Job drawing, mm, ordinate dimensions from the low corner. One solid piece. Round coordinates to 2 decimals unless told otherwise and drop trailing zeros. Order: outer loops, then holes, each group sorted by start corner. A loop starts at its lowest first (then second) coordinate and runs counter-clockwise, first axis right, second up. Notation, with made-up numbers: (-35.75, 55.25) -> (-19.75, 55.25) arc R26 cw to (-19.75, 87.25) -> close; hole circle Ø11 at (-3, 30.5). An arc over 180 degrees is marked (long way). Answer as a JSON object with one key per item and string values. Group by question number.
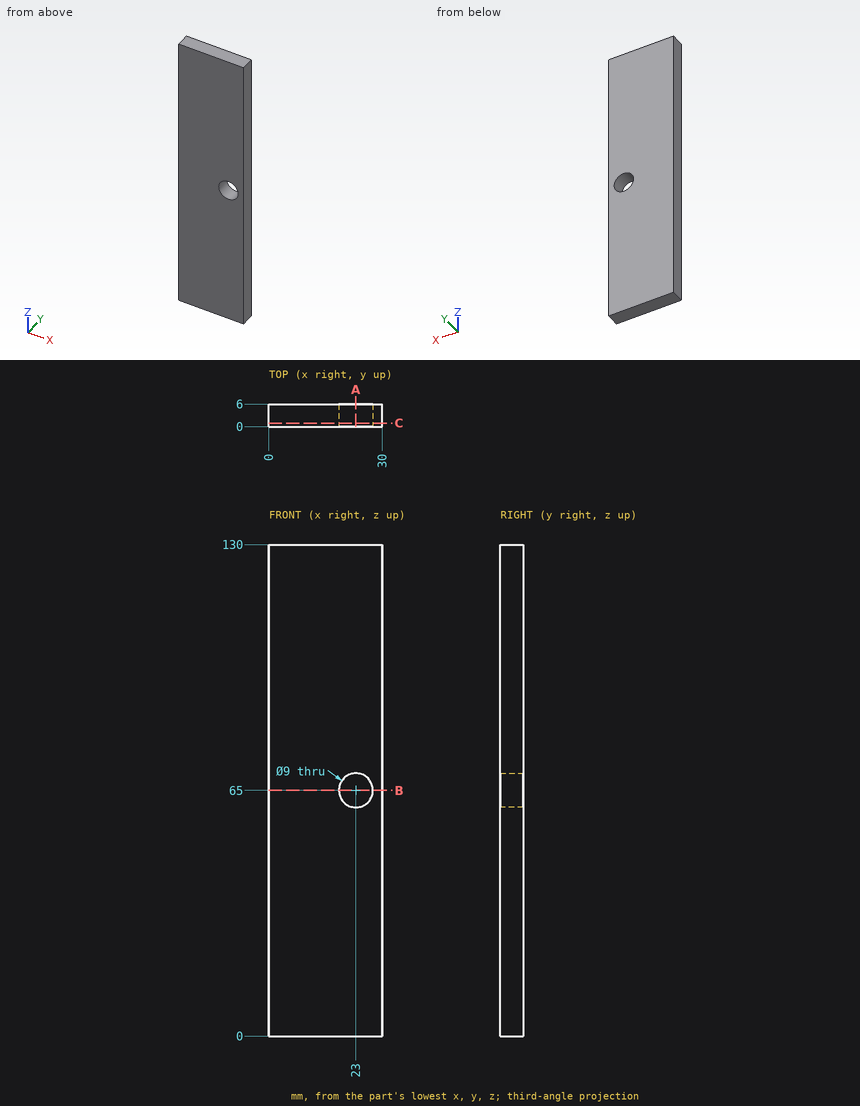
Q1. Band-saw the part on C-C (y = 0.95). List the corners of the cut face in (x, z).
Q2. Wall check: line 1 (X direction, y = 2.5, z = 65); line 2 (Z direction, x = 23, y = 3.25); line 3 (Z direction, x = 26.75, y = 5.6). Give the ranges that are in metal, low to high. Write a range as [from, to].
Q3. Band-saw the part on A-A (x = 23). List the corners of the cut face in (y, z), plus the area to 3 significant figures.
Q4. Band-saw the part on B-B (z = 65). List the corners of the cut face in (x, y), plus the area to 3 significant figures.
Completed:
{
 "1": {"outline": "(0, 0) -> (30, 0) -> (30, 130) -> (0, 130) -> close; hole circle Ø9 at (23, 65)"},
 "2": {"line 1": "[0, 18.5], [27.5, 30]", "line 2": "[0, 60.5], [69.5, 130]", "line 3": "[0, 62.51], [67.49, 130]"},
 "3": {"outline": "(0, 0) -> (6, 0) -> (6, 60.5) -> (0, 60.5) -> close; (0, 69.5) -> (6, 69.5) -> (6, 130) -> (0, 130) -> close", "area": "726 mm2"},
 "4": {"outline": "(0, 0) -> (18.5, 0) -> (18.5, 6) -> (0, 6) -> close; (27.5, 0) -> (30, 0) -> (30, 6) -> (27.5, 6) -> close", "area": "126 mm2"}
}
